Build history of the part. All positions in model axes, mm. Give positions to 0.01 mm unless a question says otherwise; leave off trailing zeros. Loops run counter-clockwise (first coordinate to the right, second up) from the corner with the lowest first, then second, coordinate; pieces in that order, holes last.
1) Band-saw the part on C-C on y = -12. List the corners of the cut face in (x, z) (3 decimals).
2) Flat gauge pin, fed straight in: P1, Ø1.5, axis at x = 4, z = 1.5, coming from the -Y side (3 decimals). Where does the tip first touch, or does it go through?
3) Wall check: line 1 (Y direction, x = 16, z = 1.3) (3 decimals); line 2 (Y direction, x = -29, z = 3); line 3 (Y direction, x = -30, z = 2.75). Give the ranges that are in metal, low to high.
4) Band-saw the part on D-D on x = 1.5. List the corners of the cut face in (y, z) (3 decimals), then the cut area to 3 significant figures.
5) Band-saw the part on B-B on x = -25.5. List the corners of the cut face in (y, z) (3 decimals), then the cut area to 3 significant figures.
6) Two-plate mould, pull along Y, no slides. Class faces 1 (the flat face through (14, 1, 0)), 2 (the cylindrical face through (-6.135, 6.882, 1.565)): +Y half, -Y half, draft (parallel to the pull), parting line (faces both ways), or undercut.
7) Band-saw the part on A-A on z = 1.2. List the corners of the cut face in (x, y) (1 decimal), then the cut area to 3 significant figures.
```python
from build123d import *

# Parameters (mm, degrees)
F1_DEPTH = 3.175


with BuildPart() as f1:
    # F0 (on Top) → F1 (new body)
    with BuildSketch(Plane.XY):
        with BuildLine():
            Line((-42.06875, -79.375), (-42.06875, -101.6))
            Line((-42.06875, -101.6), (-14.022917, -101.6))
            Line((-14.022917, -101.6), (-13.768917, -101.6))
            Line((-13.768917, -101.6), (-8.05815, -101.6))
            Line((-8.05815, -101.6), (-8.05815, -98.425))
            Line((-8.05815, -98.425), (4.64185, -98.425))
            Line((4.64185, -98.425), (17.34185, -98.425))
            Line((17.34185, -98.425), (17.34185, -101.6))
            Line((17.34185, -101.6), (50.33645, -101.6))
            Line((50.33645, -101.6), (51.35245, -101.6))
            Line((51.35245, -101.6), (51.35245, 101.6))
            Line((51.35245, 101.6), (24.579512, 101.6))
            Line((24.579512, 101.6), (17.34185, 101.6))
            Line((17.34185, 101.6), (17.34185, 98.425))
            Line((17.34185, 98.425), (4.64185, 98.425))
            Line((4.64185, 98.425), (-8.05815, 98.425))
            Line((-8.05815, 98.425), (-8.05815, 101.6))
            Line((-8.05815, 101.6), (-13.768917, 101.6))
            Line((-13.768917, 101.6), (-14.022917, 101.6))
            Line((-14.022917, 101.6), (-42.06875, 101.6))
            Line((-42.06875, 101.6), (-42.06875, 90.4875))
            ThreePointArc((-42.06875, 90.4875), (-6.127735, 5.55625), (-42.06875, -79.375))
        make_face()
    extrude(amount=F1_DEPTH)


solid = f1.part
```
Findings below:
1. outline: (-7.437, 0) - (51.352, 0) - (51.352, 3.175) - (-7.437, 3.175) - close
2. P1: stops at y = -98.425
3. line 1: y = -98.425 to 98.425
3. line 2: y = -101.6 to -64.37, 75.48 to 101.6
3. line 3: y = -101.6 to -65.71, 76.83 to 101.6
4. outline: (-98.425, 0) - (98.425, 0) - (98.425, 3.175) - (-98.425, 3.175) - close
4. area: 625 mm2
5. outline: (-101.6, 0) - (-59.32, 0) - (-59.32, 3.175) - (-101.6, 3.175) - close; (70.433, 0) - (101.6, 0) - (101.6, 3.175) - (70.433, 3.175) - close
5. area: 233 mm2
6. face 1: draft
6. face 2: undercut
7. outline: (-42.1, -101.6) - (-8.1, -101.6) - (-8.1, -98.4) - (17.3, -98.4) - (17.3, -101.6) - (51.4, -101.6) - (51.4, 101.6) - (17.3, 101.6) - (17.3, 98.4) - (-8.1, 98.4) - (-8.1, 101.6) - (-42.1, 101.6) - (-42.1, 90.5) arc R118.3 cw to (-42.1, -79.4) - close
7. area: 14,600 mm2
